from build123d import *

# Parameters (mm, degrees)
ESBO_O1_W                          = 100
ESBO_O1_H                          = 93
RESSALTO_EXTRUS_O1_DEPTH           = 6
FILETE1_R                          = 10
FILETE2_R                          = 3
ESBO_O2_W                          = 85
ESBO_O2_H                          = 20.1
CORTE_EXTRUS_O1_DEPTH              = 2
CORTE_EXTRUS_O6_REACH              = 70.398
ESBO_O8_R                          = 1.75
ESBO_O5_W                          = 8.05
ESBO_O5_H                          = 29.05
CORTE_EXTRUS_O3_DEPTH              = 2
CORTE_EXTRUS_O10_REACH             = 70.398
ESBO_O13_R                         = 1.75
ESBO_O14_R                         = 3.25
CORTE_EXTRUS_O11_DEPTH             = 2
ESBO_O6_W                          = 22.94
ESBO_O6_H                          = 15.94
CORTE_EXTRUS_O4_DEPTH              = 2
CORTE_EXTRUS_O12_REACH             = 70.398
ESBO_O15_R                         = 1.75
ESBO_O16_R                         = 3.25
CORTE_EXTRUS_O13_DEPTH             = 2
ESBO_O7_W                          = 18.71
ESBO_O7_H                          = 11.71
CORTE_EXTRUS_O5_DEPTH              = 2
CORTE_EXTRUS_O8_REACH              = 70.398
ESBO_O11_R                         = 1.75
ESBO_O12_R                         = 3.25
CORTE_EXTRUS_O9_DEPTH              = 2
ESBO_O17_W                         = 13
ESBO_O17_H                         = 35
CORTE_EXTRUS_O14_DEPTH             = 2
CORTE_EXTRUS_O15_REACH             = 70.398
ESBO_O18_R                         = 1.75
CORTE_EXTRUS_O15_DIRECTION_2_DEPTH = 69.397734022
ESBO_O19_R                         = 3.25
CORTE_EXTRUS_O18_DEPTH             = 2
CORTE_EXTRUS_O17_REACH             = 70.544
ESBO_O20_W                         = 9.4
ESBO_O20_H                         = 35
CORTE_EXTRUS_O19_REACH             = 70.544
ESBO_O21_W                         = 15
ESBO_O21_H                         = 15
FILETE3_R                          = 2
CORTE_EXTRUS_O20_REACH             = 70.544
ESBO_O22_R                         = 1.75
CORTE_EXTRUS_O21_REACH             = 70.544
ESBO_O23_R                         = 1.75


with BuildPart() as part:
    # Esboço1 → Ressalto-extrusão1 (new body)
    with BuildSketch(Plane(origin=(0, 0, 0), x_dir=(1, 0, 0), z_dir=(0, 1, 0))):
        Rectangle(ESBO_O1_W, ESBO_O1_H)
    extrude(amount=RESSALTO_EXTRUS_O1_DEPTH)

    # Filete1
    filete1_edges = [part.edges().sort_by_distance(p)[0] for p in [
        (50, 3, 46.5),
        (-50, 3, 46.5),
        (-50, 3, -46.5),
        (50, 3, -46.5),
    ]]
    fillet(filete1_edges, radius=FILETE1_R)

    # Filete2
    filete2_edges = [part.edges().sort_by_distance(p)[0] for p in [
        (0, 6, -46.5),
        (50, 6, 0),
        (-50, 6, 0),
        (0, 6, 46.5),
        (-47.071067812, 6, -43.571067812),
        (-47.071067812, 6, 43.571067812),
        (47.071067812, 6, 43.571067812),
        (47.071067812, 6, -43.571067812),
    ]]
    fillet(filete2_edges, radius=FILETE2_R)

    # Esboço2 → Corte-extrusão1 (cut)
    with BuildSketch(Plane(origin=(0, 6, 0), x_dir=(1, 0, 0), z_dir=(0, 1, 0))):
        with Locations((0, -34.45)):
            Rectangle(ESBO_O2_W, ESBO_O2_H)
    extrude(amount=-CORTE_EXTRUS_O1_DEPTH, mode=Mode.SUBTRACT)

    # Esboço8 → Corte-extrusão6 (cut, up to next)
    with BuildSketch(Plane(origin=(0, 4, 0), x_dir=(1, 0, 0), z_dir=(0, 1, 0)), mode=Mode.PRIVATE) as corte_extrus_o6_sk1:
        with Locations(Location((34.5, -29.4, 0), (0, 0, 270))):
            Circle(ESBO_O8_R)
    corte_extrus_o6_tool1 = extrude(corte_extrus_o6_sk1.sketch, amount=-CORTE_EXTRUS_O6_REACH, mode=Mode.PRIVATE) & part.part
    # Esboço8 → Corte-extrusão6 (cut, up to next)
    with BuildSketch(Plane(origin=(0, 4, 0), x_dir=(1, 0, 0), z_dir=(0, 1, 0)), mode=Mode.PRIVATE) as corte_extrus_o6_sk2:
        with Locations(Location((-34.5, -29.4, 0), (0, 0, 270))):
            Circle(ESBO_O8_R)
    corte_extrus_o6_tool2 = extrude(corte_extrus_o6_sk2.sketch, amount=-CORTE_EXTRUS_O6_REACH, mode=Mode.PRIVATE) & part.part
    add(corte_extrus_o6_tool1.solids().sort_by_distance((34.5, 4, 29.4))[0], mode=Mode.SUBTRACT)
    add(corte_extrus_o6_tool2.solids().sort_by_distance((-34.5, 4, 29.4))[0], mode=Mode.SUBTRACT)

    # Esboço5 → Corte-extrusão3 (cut)
    with BuildSketch(Plane(origin=(0, 6, 0), x_dir=(1, 0, 0), z_dir=(0, 1, 0))):
        with Locations((-39.3, 13)):
            Rectangle(ESBO_O5_W, ESBO_O5_H)
    extrude(amount=-CORTE_EXTRUS_O3_DEPTH, mode=Mode.SUBTRACT)

    # Esboço13 → Corte-extrusão10 (cut, up to next)
    with BuildSketch(Plane(origin=(0, 4, 0), x_dir=(1, 0, 0), z_dir=(0, 1, 0)), mode=Mode.PRIVATE) as corte_extrus_o10_sk1:
        with Locations(Location((-39.3, 24.025, 0), (0, 0, 270))):
            Circle(ESBO_O13_R)
    corte_extrus_o10_tool1 = extrude(corte_extrus_o10_sk1.sketch, amount=-CORTE_EXTRUS_O10_REACH, mode=Mode.PRIVATE) & part.part
    # Esboço13 → Corte-extrusão10 (cut, up to next)
    with BuildSketch(Plane(origin=(0, 4, 0), x_dir=(1, 0, 0), z_dir=(0, 1, 0)), mode=Mode.PRIVATE) as corte_extrus_o10_sk2:
        with Locations(Location((-39.3, 1.975, 0), (0, 0, 270))):
            Circle(ESBO_O13_R)
    corte_extrus_o10_tool2 = extrude(corte_extrus_o10_sk2.sketch, amount=-CORTE_EXTRUS_O10_REACH, mode=Mode.PRIVATE) & part.part
    add(corte_extrus_o10_tool1.solids().sort_by_distance((-39.3, 4, -24.025))[0], mode=Mode.SUBTRACT)
    add(corte_extrus_o10_tool2.solids().sort_by_distance((-39.3, 4, -1.975))[0], mode=Mode.SUBTRACT)

    # Esboço14 → Corte-extrusão11 (cut)
    with BuildSketch(Plane.XZ):
        with Locations(Location((-39.3, -1.975, 0), (0, 0, 270))):
            Circle(ESBO_O14_R)
        with Locations(Location((-39.3, -24.025, 0), (0, 0, 270))):
            Circle(ESBO_O14_R)
    extrude(amount=-CORTE_EXTRUS_O11_DEPTH, mode=Mode.SUBTRACT)

    # Esboço6 → Corte-extrusão4 (cut)
    with BuildSketch(Plane(origin=(0, 6, 0), x_dir=(1, 0, 0), z_dir=(0, 1, 0))):
        with Locations((27.18, 30.03)):
            Rectangle(ESBO_O6_W, ESBO_O6_H)
    extrude(amount=-CORTE_EXTRUS_O4_DEPTH, mode=Mode.SUBTRACT)

    # Esboço15 → Corte-extrusão12 (cut, up to next)
    with BuildSketch(Plane(origin=(0, 4, 0), x_dir=(1, 0, 0), z_dir=(0, 1, 0)), mode=Mode.PRIVATE) as corte_extrus_o12_sk1:
        with Locations(Location((19.21, 30.03, 0), (0, 0, 270))):
            Circle(ESBO_O15_R)
    corte_extrus_o12_tool1 = extrude(corte_extrus_o12_sk1.sketch, amount=-CORTE_EXTRUS_O12_REACH, mode=Mode.PRIVATE) & part.part
    # Esboço15 → Corte-extrusão12 (cut, up to next)
    with BuildSketch(Plane(origin=(0, 4, 0), x_dir=(1, 0, 0), z_dir=(0, 1, 0)), mode=Mode.PRIVATE) as corte_extrus_o12_sk2:
        with Locations(Location((35.15, 30.03, 0), (0, 0, 270))):
            Circle(ESBO_O15_R)
    corte_extrus_o12_tool2 = extrude(corte_extrus_o12_sk2.sketch, amount=-CORTE_EXTRUS_O12_REACH, mode=Mode.PRIVATE) & part.part
    add(corte_extrus_o12_tool1.solids().sort_by_distance((19.21, 4, -30.03))[0], mode=Mode.SUBTRACT)
    add(corte_extrus_o12_tool2.solids().sort_by_distance((35.15, 4, -30.03))[0], mode=Mode.SUBTRACT)

    # Esboço16 → Corte-extrusão13 (cut)
    with BuildSketch(Plane.XZ):
        with Locations(Location((19.21, -30.03, 0), (0, 0, 270))):
            Circle(ESBO_O16_R)
        with Locations(Location((35.15, -30.03, 0), (0, 0, 270))):
            Circle(ESBO_O16_R)
    extrude(amount=-CORTE_EXTRUS_O13_DEPTH, mode=Mode.SUBTRACT)

    # Esboço7 → Corte-extrusão5 (cut)
    with BuildSketch(Plane(origin=(0, 6, 0), x_dir=(1, 0, 0), z_dir=(0, 1, 0))):
        with Locations((32.22, 11.9)):
            Rectangle(ESBO_O7_W, ESBO_O7_H)
    extrude(amount=-CORTE_EXTRUS_O5_DEPTH, mode=Mode.SUBTRACT)

    # Esboço11 → Corte-extrusão8 (cut, up to next)
    with BuildSketch(Plane(origin=(0, 4, 0), x_dir=(1, 0, 0), z_dir=(0, 1, 0)), mode=Mode.PRIVATE) as corte_extrus_o8_sk1:
        with Locations(Location((26.365, 11.9, 0), (0, 0, 270))):
            Circle(ESBO_O11_R)
    corte_extrus_o8_tool1 = extrude(corte_extrus_o8_sk1.sketch, amount=-CORTE_EXTRUS_O8_REACH, mode=Mode.PRIVATE) & part.part
    # Esboço11 → Corte-extrusão8 (cut, up to next)
    with BuildSketch(Plane(origin=(0, 4, 0), x_dir=(1, 0, 0), z_dir=(0, 1, 0)), mode=Mode.PRIVATE) as corte_extrus_o8_sk2:
        with Locations(Location((38.075, 11.9, 0), (0, 0, 270))):
            Circle(ESBO_O11_R)
    corte_extrus_o8_tool2 = extrude(corte_extrus_o8_sk2.sketch, amount=-CORTE_EXTRUS_O8_REACH, mode=Mode.PRIVATE) & part.part
    add(corte_extrus_o8_tool1.solids().sort_by_distance((26.365, 4, -11.9))[0], mode=Mode.SUBTRACT)
    add(corte_extrus_o8_tool2.solids().sort_by_distance((38.075, 4, -11.9))[0], mode=Mode.SUBTRACT)

    # Esboço12 → Corte-extrusão9 (cut)
    with BuildSketch(Plane.XZ):
        with Locations(Location((26.365, -11.9, 0), (0, 0, 270))):
            Circle(ESBO_O12_R)
        with Locations(Location((38.075, -11.9, 0), (0, 0, 270))):
            Circle(ESBO_O12_R)
    extrude(amount=-CORTE_EXTRUS_O9_DEPTH, mode=Mode.SUBTRACT)

    # Esboço17 → Corte-extrusão14 (cut)
    with BuildSketch(Plane(origin=(0, 6, 0), x_dir=(1, 0, 0), z_dir=(0, 1, 0))):
        with Locations((-18.77, -0.27)):
            Rectangle(ESBO_O17_W, ESBO_O17_H)
    extrude(amount=-CORTE_EXTRUS_O14_DEPTH, mode=Mode.SUBTRACT)

    # Esboço18 → Corte-extrusão15 (cut, up to next)
    with BuildSketch(Plane(origin=(0, 4, 0), x_dir=(1, 0, 0), z_dir=(0, 1, 0)), mode=Mode.PRIVATE) as corte_extrus_o15_sk1:
        with Locations(Location((-21.77, 13.73, 0), (0, 0, 90))):
            Circle(ESBO_O18_R)
    corte_extrus_o15_tool1 = extrude(corte_extrus_o15_sk1.sketch, amount=-CORTE_EXTRUS_O15_REACH, mode=Mode.PRIVATE) & part.part
    # Esboço18 → Corte-extrusão15 (cut, up to next)
    with BuildSketch(Plane(origin=(0, 4, 0), x_dir=(1, 0, 0), z_dir=(0, 1, 0)), mode=Mode.PRIVATE) as corte_extrus_o15_sk2:
        with Locations(Location((-21.77, -14.27, 0), (0, 0, 90))):
            Circle(ESBO_O18_R)
    corte_extrus_o15_tool2 = extrude(corte_extrus_o15_sk2.sketch, amount=-CORTE_EXTRUS_O15_REACH, mode=Mode.PRIVATE) & part.part
    add(corte_extrus_o15_tool1.solids().sort_by_distance((-21.77, 4, -13.73))[0], mode=Mode.SUBTRACT)
    add(corte_extrus_o15_tool2.solids().sort_by_distance((-21.77, 4, 14.27))[0], mode=Mode.SUBTRACT)

    # Esboço18 → Corte-extrusão15 direction 2 (cut)
    with BuildSketch(Plane(origin=(0, 4, 0), x_dir=(1, 0, 0), z_dir=(0, 1, 0))):
        with Locations(Location((-21.77, 13.73, 0), (0, 0, 90))):
            Circle(ESBO_O18_R)
        with Locations(Location((-21.77, -14.27, 0), (0, 0, 90))):
            Circle(ESBO_O18_R)
    extrude(amount=CORTE_EXTRUS_O15_DIRECTION_2_DEPTH, mode=Mode.SUBTRACT)

    # Esboço19 → Corte-extrusão18 (cut)
    with BuildSketch(Plane.XZ):
        with Locations(Location((-21.77, 14.27, 0), (0, 0, 270))):
            Circle(ESBO_O19_R)
        with Locations(Location((-21.77, -13.73, 0), (0, 0, 270))):
            Circle(ESBO_O19_R)
    extrude(amount=-CORTE_EXTRUS_O18_DEPTH, mode=Mode.SUBTRACT)

    # Esboço20 → Corte-extrusão17 (cut, up to next)
    with BuildSketch(Plane(origin=(0, 6, 0), x_dir=(1, 0, 0), z_dir=(0, 1, 0)), mode=Mode.PRIVATE) as corte_extrus_o17_sk1:
        with Locations((-0.8, -4.9)):
            Rectangle(ESBO_O20_W, ESBO_O20_H)
    corte_extrus_o17_tool1 = extrude(corte_extrus_o17_sk1.sketch, amount=-CORTE_EXTRUS_O17_REACH, mode=Mode.PRIVATE) & part.part
    add(corte_extrus_o17_tool1.solids().sort_by_distance((-0.8, 6, 4.9))[0], mode=Mode.SUBTRACT)

    # Esboço21 → Corte-extrusão19 (cut, up to next)
    with BuildSketch(Plane(origin=(0, 6, 0), x_dir=(1, 0, 0), z_dir=(0, 1, 0)), mode=Mode.PRIVATE) as corte_extrus_o19_sk1:
        with Locations((0, 32.5)):
            Rectangle(ESBO_O21_W, ESBO_O21_H)
    corte_extrus_o19_tool1 = extrude(corte_extrus_o19_sk1.sketch, amount=-CORTE_EXTRUS_O19_REACH, mode=Mode.PRIVATE) & part.part
    add(corte_extrus_o19_tool1.solids().sort_by_distance((0, 6, -32.5))[0], mode=Mode.SUBTRACT)

    # Filete3
    filete3_edges = [part.edges().sort_by_distance(p)[0] for p in [
        (-5.5, 3, 22.4),
        (-5.5, 3, -12.6),
        (3.9, 3, -12.6),
        (3.9, 3, 22.4),
        (-7.5, 3, -25),
        (-7.5, 3, -40),
        (7.5, 3, -40),
        (7.5, 3, -25),
    ]]
    fillet(filete3_edges, radius=FILETE3_R)

    # Esboço22 → Corte-extrusão20 (cut, up to next)
    with BuildSketch(Plane(origin=(0, 6, 0), x_dir=(1, 0, 0), z_dir=(0, 1, 0)), mode=Mode.PRIVATE) as corte_extrus_o20_sk1:
        with Locations(Location((41, -18.4, 0), (0, 0, 270))):
            Circle(ESBO_O22_R)
    corte_extrus_o20_tool1 = extrude(corte_extrus_o20_sk1.sketch, amount=-CORTE_EXTRUS_O20_REACH, mode=Mode.PRIVATE) & part.part
    corte_extrus_o20 = corte_extrus_o20_tool1.solids().sort_by_distance((41, 6, 18.4))[0]
    add(corte_extrus_o20, mode=Mode.SUBTRACT)

    # Esboço23 → Corte-extrusão21 (cut, up to next)
    with BuildSketch(Plane(origin=(0, 6, 0), x_dir=(1, 0, 0), z_dir=(0, 1, 0)), mode=Mode.PRIVATE) as corte_extrus_o21_sk1:
        with Locations(Location((42, 38.5, 0), (0, 0, 270))):
            Circle(ESBO_O23_R)
    corte_extrus_o21_tool1 = extrude(corte_extrus_o21_sk1.sketch, amount=-CORTE_EXTRUS_O21_REACH, mode=Mode.PRIVATE) & part.part
    corte_extrus_o21 = corte_extrus_o21_tool1.solids().sort_by_distance((42, 6, -38.5))[0]
    add(corte_extrus_o21, mode=Mode.SUBTRACT)

    # Espelhar1: Corte-extrusão20, Corte-extrusão21 across plane
    add(corte_extrus_o20.mirror(Plane(origin=(0, 0, 0), x_dir=(0, 0, 1), z_dir=(1, 0, 0))), mode=Mode.SUBTRACT)
    add(corte_extrus_o21.mirror(Plane(origin=(0, 0, 0), x_dir=(0, 0, 1), z_dir=(1, 0, 0))), mode=Mode.SUBTRACT)


solid = part.part
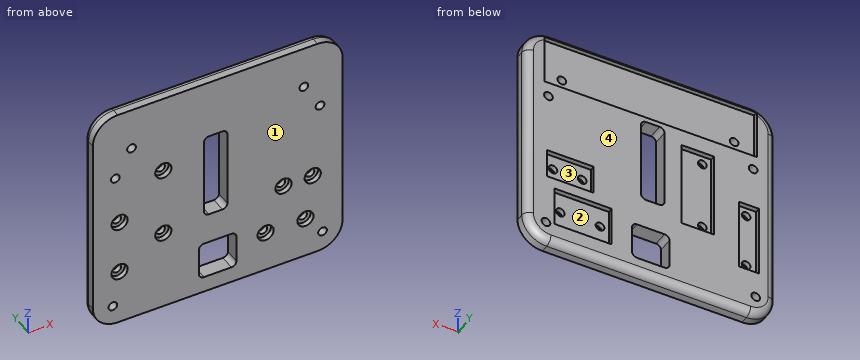
Can you work these out from the model? Positions are in its coordinate system, mm. Face numbers are marked on the shaded views. A direction names the side the tool comes from. Coordinates: 2 decimals unless noted, no trailing zeros. Loops run counter-clockwise (first coordinate to the right, second up) from the corner with the lowest first, then second, coordinate; pieces in that order, holes last. Notation, with made-up numbers: (-32.5, 70) - (4.5, 70) arc R20 ccw to (4.5, 99) - close; hole circle Ø10 at (9, -2). An arc over 180 degrees is marked (long way). Answer as a JSON object with one key per item and string values. Group by question number.
Item 1: On a 3-axis mill with a long thin cutter (end or side, diameter ignored), from which of +Z, -Z, +X, -X, +Y, -Y can I reach the whole of each face in a straight line? I mean the marked faces 1 and 2. Say none if no direction works.
Item 2: If we section it at C-C (x = -16.5): List the corners of the cut face in (y, z) for me.
Item 3: If we section it at B-B (z = -29.5): State how many separate pieces and enclosed holes the cut face has, plus the area to 3 significant figures.
Item 4: For pin 1 (4.5 mm diameter, centred on x = 38.075, z = -11.9, fed in from -Y); pin 2 (1 mm diameter, centred on y = 4.5, z = 9, fed in from +X); pin 3 (1.5 mm diameter, centred on x = -22, y = 4.5, fed in from +Z); pin 4 (10 mm diameter, centred on x = -36, z = -20, fed in from -Y), each with a flat end and sliding along its axis, tell me the tip position at first contact or that it passes through.
Item 5: If I drill on L1, parallel to X at y = 2, z = -5.5; L2, parallel to X at y = 5.5, z = 20; L3, parallel to X at y = 5.5, z = -11 (3 decimals), over which ranges is the centre line in solid material (lowest first)? Write a range as from..to.
Item 6: If we section it at A-A (x = 19.21): List the corners of the cut face in (y, z) for me, plus the area to 3 significant figures.
Item 7: If we mould it in two halves opening along X, with no side actions, what happens to the marked faces 3 and 4? For each: released by +X, released by -X, zero draft, split by the parting line, or undercut.
Returned:
{
 "1": {"face 1": "+Z, -Z, +X, -X, -Y", "face 2": "+Y"},
 "2": {"outline": "(0, -46.5) - (3, -46.5) arc R3 ccw to (6, -43.5) - (6, -17.23) - (4, -17.23) - (4, 17.77) - (6, 17.77) - (6, 24.4) - (4, 24.4) - (4, 44.5) - (5.83, 44.5) arc R3 ccw to (3, 46.5) - (0, 46.5) - close"},
 "3": {"separate pieces": "4", "enclosed holes": "0", "area": "421 mm²"},
 "4": {"pin 1": "stops at y = 2", "pin 2": "stops at x = 49.83", "pin 3": "stops at z = 46.4", "pin 4": "stops at y = 0"},
 "5": {"L1": "x = -50..-5.5, 3.9..50", "L2": "x = -48.66..-41.71, -40.29..-5.5, 3.9..40.29, 41.71..48.66", "L3": "x = -48.658..-43.325, -35.275..-25.27, -12.27..-5.46, 3.86..22.865, 41.575..48.658"},
 "6": {"outline": "(0, -46.5) - (3, -46.5) arc R3 ccw to (6, -43.5) - (6, -38) - (4, -38) - (4, -31.78) - (2, -31.78) - (2, -33.28) - (0, -33.28) - close; (0, -26.78) - (2, -26.78) - (2, -28.28) - (4, -28.28) - (4, -22.06) - (6, -22.06) - (6, 24.4) - (4, 24.4) - (4, 44.5) - (5.83, 44.5) arc R3 ccw to (3, 46.5) - (0, 46.5) - close", "area": "462 mm²"},
 "7": {"face 3": "undercut", "face 4": "zero draft"}
}
